Geometry: final body of the model. Coordinates: model frame, mm. A direction names the side the tool comes from. Round coordinates to 2 decimals unless told otherwise and drop trailing zeros. Loops run counter-clockwise (first coordinate to the right, second up) from the corner with the lowest first, then second, coordinate; pieces in that order, holes last. Notation, with made-up numbers: (-16, -18) -> (10, -18) arc R28 cw to (10, 15) -> close; hole circle Ø1 at (42, -18.75). An arc over 180 degrees is marked (long way). Answer in a Markdown table with one row per item.
```python
from build123d import *

# Parameters (mm, degrees)
SKETCH_1_W          = 10
SKETCH_1_H          = 30
SKETCH_1_R          = 1.6
EXTRUDE_1_DEPTH     = 3
SKETCH_5_R          = 1.6
SKETCH_5_W          = 10
SKETCH_5_H          = 3
EXTRUDE_4_DEPTH     = 3
SKETCH_6_R          = 1
CUT_EXTRUDE_1_DEPTH = 35.073450075
FILLET_1_R          = 2


with BuildPart() as part:
    # 草图1 → 凸台-拉伸1 (new body)
    with BuildSketch(Plane(origin=(0, 0, 0), x_dir=(1, 0, 0), z_dir=(0, 1, 0))):
        Rectangle(SKETCH_1_W, SKETCH_1_H)
        with Locations(Location((0, 0, 0), (0, 0, 270))):
            Circle(SKETCH_1_R, mode=Mode.SUBTRACT)
        with Locations(Location((0, 10, 0), (0, 0, 270))):
            Circle(SKETCH_1_R, mode=Mode.SUBTRACT)
        with Locations(Location((0, -10, 0), (0, 0, 90))):
            Circle(SKETCH_1_R, mode=Mode.SUBTRACT)
    extrude(amount=EXTRUDE_1_DEPTH)

    # 草图5 → 凸台-拉伸4 (add)
    with BuildSketch(Plane.XZ):
        with BuildLine():
            Line((24, -13), (24, -24))
            Line((24, -24), (8, -24))
            Line((8, -24), (8, -15))
            Line((8, -15), (5, -15))
            Line((5, -15), (5, 5.196152423))
            ThreePointArc((5, 5.196152423), (6, 3.464101615), (8, 3.464101615))
            ThreePointArc((8, 3.464101615), (13.127799472, 2.493365288), (12.931173967, -2.721804397))
            Line((12.931173967, -2.721804397), (24, -13))
        make_face()
        with Locations(Location((10, 0, 0), (0, 0, 270))):
            Circle(SKETCH_5_R, mode=Mode.SUBTRACT)
        with Locations((16, -19.5)):
            Rectangle(SKETCH_5_W, SKETCH_5_H, mode=Mode.SUBTRACT)
    extrude(amount=-EXTRUDE_4_DEPTH)

    # 草图6 → 切除-拉伸1 (cut, through all)
    with BuildSketch(Plane.XZ):
        with Locations((20.072975189, -18.375)):
            Circle(SKETCH_6_R)
        with Locations((11.927024811, -18.375)):
            Circle(SKETCH_6_R)
        with Locations((11.927024811, -20.625)):
            Circle(SKETCH_6_R)
        with Locations((20.072975189, -20.625)):
            Circle(SKETCH_6_R)
        with Locations((7, -15)):
            Circle(SKETCH_6_R)
    extrude(amount=-CUT_EXTRUDE_1_DEPTH, mode=Mode.SUBTRACT)

    # 圆角1
    fillet_1_edges = [part.edges().sort_by_distance(p)[0] for p in [
        (8, 1.5, -24),
        (24, 1.5, -24),
        (24, 1.5, -13),
        (12.931173967, 1.5, -2.721804397),
        (5, 1.5, 15),
        (-5, 1.5, 15),
        (-5, 1.5, -15),
    ]]
    fillet(fillet_1_edges, radius=FILLET_1_R)


solid = part.part
```
Item 1: First-contact query: P1, Ø2.5, axis at x = 0, z = 0, coming from the +Y side; P2, Ø3, axis at x = 13.5, z = -6.5, coming from the -Y side; P3, Ø0.9, axis at x = 1, y = 1.5, coming from the -Z side; P4, Ø0.9, axis at y = 1.5, z = 8, coming from the +X side. Flat tips, straight axial feed; report the tip coordinate or a pass-through.
Ans:
| item | result |
|---|---|
| P1 | through |
| P2 | y = 0 |
| P3 | z = -15 |
| P4 | x = 5 |
Item 2: Section query B-B, the plane x = 0. Output: boundary loops of the cut face in (y, z), and give its area (3 significant figures).
Ans:
| item | result |
|---|---|
| outline | (0, -15) -> (3, -15) -> (3, -11.6) -> (0, -11.6) -> close; (0, -8.4) -> (3, -8.4) -> (3, -1.6) -> (0, -1.6) -> close; (0, 1.6) -> (3, 1.6) -> (3, 8.4) -> (0, 8.4) -> close; (0, 11.6) -> (3, 11.6) -> (3, 15) -> (0, 15) -> close |
| area | 61.2 mm2 |
Item 3: Section query A-A, the plane z = 0. Output: boundary loops of the cut face in (x, y).
Ans:
| item | result |
|---|---|
| outline | (-5, 0) -> (-1.6, 0) -> (-1.6, 3) -> (-5, 3) -> close; (1.6, 0) -> (8.4, 0) -> (8.4, 3) -> (1.6, 3) -> close; (11.6, 0) -> (14, 0) -> (14, 3) -> (11.6, 3) -> close |
Item 4: Ray query, L1, parallel to X at y = 0.9, z = 0; L2, parallel to X at y = 1.45, z = -18.5; L3, parallel to X at y = 2.2, z = -10. Return the intervals inside material, ascending.
Ans:
| item | result |
|---|---|
| L1 | -5 to -1.6, 1.6 to 8.4, 11.6 to 14 |
| L2 | 8 to 10.93, 21.07 to 24 |
| L3 | -5 to -1.6, 1.6 to 20.77 |
Item 5: Mould query, pull axis X, two halves, no side actions, for faces 4 (the cylindrical face through (23.43, 1.52, -23.4)), 5 (the cylindrical face through (8.44, 1.48, 0.35)), 6 (the flat face through (16, 1, -24)). Classes: released by +X, released by -X, zero draft, split by the parting line, or undercut.
Ans:
| item | result |
|---|---|
| face 4 | released by +X |
| face 5 | undercut |
| face 6 | zero draft |
Item 6: Section query D-D, the plane x = 20.25. Output: boundary loops of the cut face in (y, z).
Ans:
| item | result |
|---|---|
| outline | (0, -24) -> (3, -24) -> (3, -21.61) -> (0, -21.61) -> close; (0, -17.39) -> (3, -17.39) -> (3, -9.52) -> (0, -9.52) -> close |
Item 7: Section query C-C, the plane z = -9. Output: boundary loops of the cut face in (x, y).
Ans:
| item | result |
|---|---|
| outline | (-5, 0) -> (-1.25, 0) -> (-1.25, 3) -> (-5, 3) -> close; (1.25, 0) -> (19.69, 0) -> (19.69, 3) -> (1.25, 3) -> close |
Item 8: Set-up query: faces 1 (the cylindrical face through (7, 1, -14)), 2 (the flat face through (21, 1, -20)), 3 (the flat face through (2, 1, -15)). Return all of +Z, -Z, +X, -X, +Y, -Y with unobstructed straight access to the full face (end or side cutting, diameter ignored); none if empty.
Ans:
| item | result |
|---|---|
| face 1 | -Z, +Y, -Y |
| face 2 | +Y, -Y |
| face 3 | -Z, -X, +Y, -Y |
